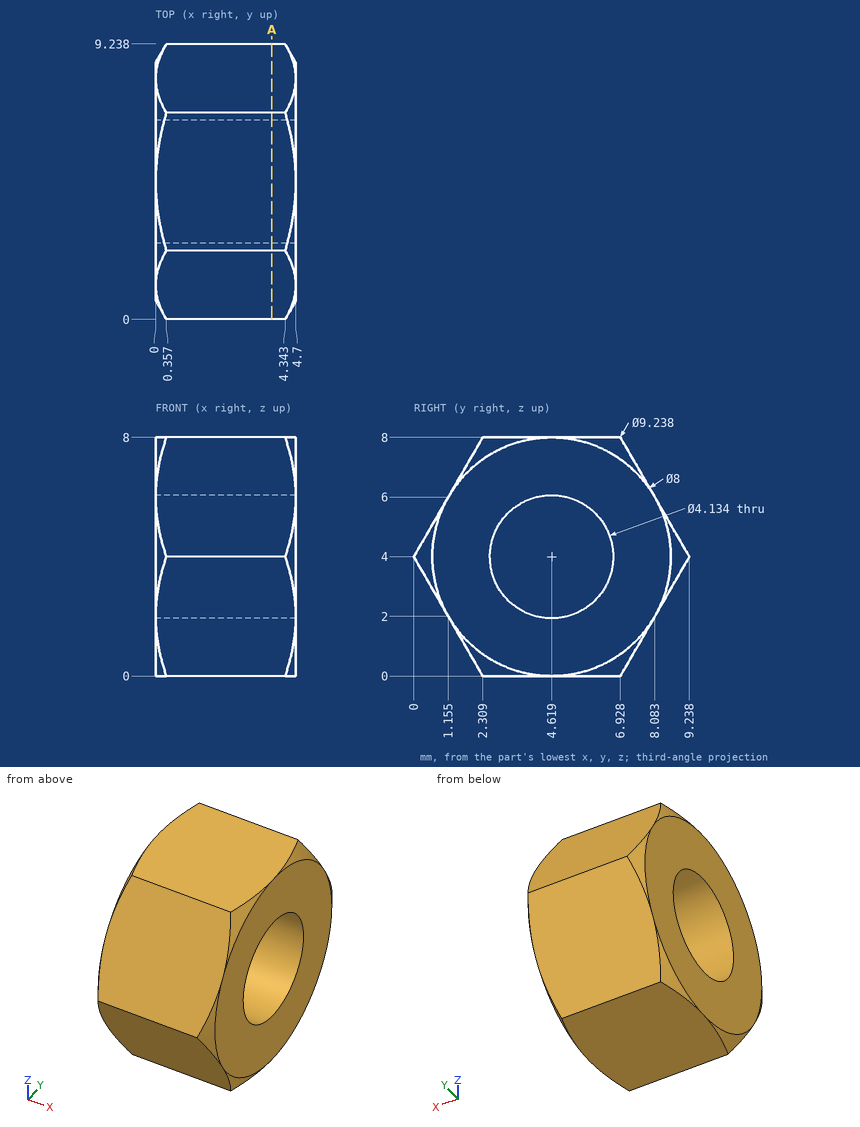
The figure shows three views and two pictorial views of one solid part (mm, origin at its lowest corner). Answer the questions. Round coordinates to 2 decimals unless told otherwise and drop trailing zeros. Write each loop counter-clockwise with the first axis right and the second up, starting at its lowest first coordinate (ties: lowest second). Pieces come first, ordered by that corner, then holes. Notation, with made-up numbers: (-12, 30) - (17, 30) arc R33 cw to (17, 63) - close; hole circle Ø9 at (-32, -23.5). An arc over 180 degrees is marked (long way). Answer in a Markdown table with one row per item. Add a question column.
1. Find the intervals of material crossed by line 1 along Z through (x, y) = (4.2, 6); line 2 along Y through (x, z) = (4.1, 5.5) (1 decimal); line 3 along Z through (x, y) = (0.6, 4), in increasing order. Write a range as from..to.
2. Given pin 1 (1 mm diameter, centred on y = 4, z = 3, fed in from -X); pin 2 (2 mm diameter, centred on x = 2, z = 6.5, fed in from +Y), each flat-ended and moving along its own axis, determine where each tip first touches the part or whether it passes through.
3. A cutting plane is placed at A-A, the plane x = 3.9. Determine the outline of the cut face in (y, z), and give its area (3 significant figures).
Worked out:
| question | item | result |
|---|---|---|
| 1 | line 1 | 0..2.46, 5.54..8 |
| 1 | line 2 | 0.9..3.2, 6..8.4 |
| 1 | line 3 | 0..2.03, 5.97..8 |
| 2 | pin 1 | through |
| 2 | pin 2 | y = 8.37 |
| 3 | outline | (0, 4) - (2.31, 0) - (6.93, 0) - (9.24, 4) - (6.93, 8) - (2.31, 8) - close; hole circle Ø4.13 at (4.62, 4) |
| 3 | area | 42.0 mm^2 |
